from build123d import *

# Parameters (mm, degrees)
SKETCH2_W           = 1200
SKETCH2_H           = 1200
BOSS_EXTRUDE1_DEPTH = 600
SHELL1_T            = -100
SKETCH3_W           = 1200
SKETCH3_H           = 1200
BOSS_EXTRUDE2_DEPTH = 100
SKETCH4_R           = 130
CUT_EXTRUDE1_DEPTH  = 601
SKETCH5_W           = 130
SKETCH5_H           = 130
CUT_EXTRUDE2_DEPTH  = 150
CIRPATTERN2_COUNT   = 4


with BuildPart() as part:
    # Sketch2 → Boss-Extrude1 (new body)
    with BuildSketch(Plane.XY):
        Rectangle(SKETCH2_W, SKETCH2_H)
    extrude(amount=BOSS_EXTRUDE1_DEPTH)

    # Shell1
    shell1_openings = [part.faces().sort_by_distance(p)[0] for p in [
        (0, 0, 600),
    ]]
    offset(amount=SHELL1_T, openings=shell1_openings, kind=Kind.INTERSECTION)

    # Sketch3 → Boss-Extrude2 (add)
    with BuildSketch(Plane.XY.offset(600)):
        Rectangle(SKETCH3_W, SKETCH3_H)
    extrude(amount=-BOSS_EXTRUDE2_DEPTH)

    # Sketch4 → Cut-Extrude1 (cut, through all)
    with BuildSketch(Plane.XY):
        Circle(SKETCH4_R)
    extrude(amount=CUT_EXTRUDE1_DEPTH, mode=Mode.SUBTRACT)

    # Sketch5 → Cut-Extrude2 (cut)
    with BuildSketch(Plane(origin=(0, 0, 0), x_dir=(-1, 0, 0), z_dir=(0, 0, -1))):
        with Locations((-310, 0)):
            Rectangle(SKETCH5_W, SKETCH5_H)
    cut_extrude2 = extrude(amount=-CUT_EXTRUDE2_DEPTH, mode=Mode.SUBTRACT)

    # CirPattern2: Cut-Extrude2 ×4 about axis
    cirpattern2_axis = Axis((0, 0, 0), (0, 0, 1))
    for i in range(1, CIRPATTERN2_COUNT):
        add(cut_extrude2.rotate(cirpattern2_axis, i * 360 / CIRPATTERN2_COUNT), mode=Mode.SUBTRACT)


solid = part.part
Verification items for the finished model (mm, model axes). A direction names the side the tool comes from. Coordinates: 2 decimals unless noted, no trailing zeros. Write each loop counter-clockwise with the first axis right and the second up, starting at its lowest first coordinate (ties: lowest second). Pieces come first, ordered by that corner, then holes. Notation, with made-up numbers: (43, -9) -> (55, -9) arc R12 cw to (55, 10) -> close; hole circle Ø2 at (57.5, -12.5). An arc over 180 degrees is marked (long way). One line per item, written item: value. Start each with the question number.
Q1. Go/stop test with a flat-tipped pin: P1, Ø12, axis at x = -0.5, y = 342.5, coming from the -Z side. Record where the tip stops, or that it passes through.
Q2. Access from +Z, -Z, +X, -X, +Y, -Y to the whole of each face (thin tool, end or side, straight path). Record for faces 1 (the flat face through (-118, 118, 100)), 2 (the flat face through (-600, -8, 296)), 3 (the flat face through (-1, -245, 49)).
Q3. Thickness scan on L1, parallel to X at y = 0, z = 38; L2, parallel to Z at x = -482.5, y = 158.5. Record the ranges inside material, lowest first. Write a range as from..to.
Q4. Mould release check, pull along Z, two halves, no side actions. Record for faces 4 (the flat face through (-8, -600, 296)), 5 (the flat face through (-8, 142, 0)), 6 (the flat face through (-500, -7, 297)): pulls with the +Z half, pulls with the -Z half, needs draft (parallel to the pull), parting line crosses it, or undercut.
Q5. Cross-section at A-A on y = 0. Enter the section's corners in (x, z).
Q6. Cross-section at D-D on y = 421. Enter the section's corners in (x, z).
Q7. Cross-section at B-B on z = 467. Enter the section's corners in (x, y), and give its area (3 significant figures).
Checked values:
1. P1: stops at z = 500
2. face 1: none
2. face 2: +Z, -Z, -X, +Y, -Y
2. face 3: -Z
3. L1: x = -600..-375, -245..-130, 130..245, 375..600
3. L2: z = 0..100, 500..600
4. face 4: needs draft
4. face 5: pulls with the -Z half
4. face 6: undercut
5. outline: (-600, 0) -> (-375, 0) -> (-375, 100) -> (-500, 100) -> (-500, 500) -> (-130, 500) -> (-130, 600) -> (-600, 600) -> close; (-245, 0) -> (-130, 0) -> (-130, 100) -> (-245, 100) -> close; (130, 0) -> (245, 0) -> (245, 100) -> (130, 100) -> close; (130, 500) -> (500, 500) -> (500, 100) -> (375, 100) -> (375, 0) -> (600, 0) -> (600, 600) -> (130, 600) -> close
6. outline: (-600, 0) -> (600, 0) -> (600, 600) -> (-600, 600) -> close; hole (-500, 100) -> (500, 100) -> (500, 500) -> (-500, 500) -> close
7. outline: (-600, -600) -> (600, -600) -> (600, 600) -> (-600, 600) -> close; hole (-500, -500) -> (500, -500) -> (500, 500) -> (-500, 500) -> close
7. area: 440,000 mm²
